```python
from build123d import *

# Parameters (mm, degrees)
SKETCH1_R           = 5
SKETCH1_R_2         = 1.740677898
BOSS_EXTRUDE1_DEPTH = 6
SKETCH2_R           = 1.25
CUT_EXTRUDE1_DEPTH  = 11


with BuildPart() as part:
    # Sketch1 → Boss-Extrude1 (new body)
    with BuildSketch(Plane.XY):
        with Locations((-35.04245283, -0.806603774)):
            Circle(SKETCH1_R)
        with Locations((-35.04245283, -0.806603774)):
            Circle(SKETCH1_R_2, mode=Mode.SUBTRACT)
        with BuildLine():
            Line((-16.04245283, 4.193396226), (-35.04245283, 4.193396226))
            ThreePointArc((-35.04245283, 4.193396226), (-31.506918924, 2.728930132), (-30.04245283, -0.806603774))
            ThreePointArc((-30.04245283, -0.806603774), (-31.506918924, -4.34213768), (-35.04245283, -5.806603774))
            Line((-35.04245283, -5.806603774), (-16.04245283, -5.806603774))
            ThreePointArc((-16.04245283, -5.806603774), (-21.04245283, -0.806603774), (-16.04245283, 4.193396226))
        make_face()
        with Locations((-16.04245283, -0.806603774)):
            Circle(SKETCH1_R)
        with Locations((-16.04245283, -0.806603774)):
            Circle(SKETCH1_R_2, mode=Mode.SUBTRACT)
    extrude(amount=BOSS_EXTRUDE1_DEPTH)

    # Sketch2 → Cut-Extrude1 (cut, through all)
    with BuildSketch(Plane(origin=(0, 4.193396226, 0), x_dir=(1, 0, 0), z_dir=(0, 1, 0))):
        with Locations((-16.04245283, -3)):
            Circle(SKETCH2_R)
    extrude(amount=-CUT_EXTRUDE1_DEPTH, mode=Mode.SUBTRACT)


solid = part.part
```
Can you work these out from the model? Positions are in its coordinate system, mm. Give positions to 0.01 mm unless a question says otherwise; leave off trailing zeros. Order: outer loops, then holes, each group sorted by start corner. A loop starts at its lowest first (then second) coordinate and runs counter-clockwise, first axis right, second up. Notation, with made-up numbers: M -28,31 L 7,31 A20 ccw 7,62 Z; hole C 22,31 d1. An arc over 180 degrees is marked long. Write item = value, one per line. Start each with the question number.
Q1. Suppose I cut it at A-A (z = 3). Write out the boundary of the cut face in (x, y), plus the area to 3 significant figures.
Q2. Suppose I cut it at B-B (x = -15.5). Write out the boundary of the cut face in (y, z), plus the area to 3 significant figures.
Q3. Suppose I cut it at D-D (y = -4.75). Write out the boundary of the cut face in (x, z).
Q4. Suppose I cut it at C-C (z = 1). Write out the boundary of the cut face in (x, y).
Q5. We'd pull the mould along X, two halves only. Please class faces 1 (the cylindrical face through (-11.044, -0.917, 2.958)), 2 (the flat face through (-25, 4.193, 3)), 3 (the cylindrical face through (-17.78, -0.73, 2.96)): pulls with the +X half, pulls with the -X half, needs draft (parallel to the pull), parting line crosses it, or undercut.
Q6. I need wall thicknesses on probe 1 along X at (y, z) = (-0.75, 4.75); probe 2 along X at (y, z) = (0.5, 3.25); probe 3 along Y at (x, z) = (-35, 5). Which ranges of each line are inside material? Lowest first, please. Write a range as [from, to].
Q7. Will these pins go through, and if not, where does the flat tip stop? pin 1 Ø2 at (y, z) = (2.5, 3.5) entering from -X; pin 2 Ø2 at (x, y) = (-35.04, -0.81) entering from -Z.
Check result:
q1.outline = M -35.04,-5.81 L -17.29,-5.81 L -17.29,-2.02 A1.74 cw -17.29,0.4 L -17.29,4.19 L -35.04,4.19 A5 ccw Z; M -14.79,-5.65 A5 ccw -14.79,4.03 L -14.79,0.4 A1.74 cw -14.79,-2.02 Z; hole C -35.04,-0.81 d3.48
q1.area = 233 mm2
q2.outline = M -5.78,0 L -2.46,0 L -2.46,1.87 L -5.78,1.87 Z; M -5.78,4.13 L -2.46,4.13 L -2.46,6 L -5.78,6 Z; M 0.85,0 L 4.16,0 L 4.16,1.87 L 0.85,1.87 Z; M 0.85,4.13 L 4.16,4.13 L 4.16,6 L 0.85,6 Z
q2.area = 24.9 mm2
q3.outline = M -38.12,0 L -12.97,0 L -12.97,6 L -38.12,6 Z; hole C -16.04,3 d2.5
q4.outline = M -35.04,-5.81 L -16.04,-5.81 A5 ccw -16.04,4.19 L -35.04,4.19 A5 ccw Z; hole C -35.04,-0.81 d3.48; hole C -16.04,-0.81 d3.48
q5.face_1 = pulls with the +X half
q5.face_2 = needs draft
q5.face_3 = undercut
q6.probe_1 = [-40.04, -36.78], [-33.3, -17.78], [-14.3, -11.04]
q6.probe_2 = [-39.87, -36.19], [-33.89, -17.27], [-14.82, -11.22]
q6.probe_3 = [-5.81, -2.55], [0.93, 4.19]
q7.pin_1 = -39.48
q7.pin_2 = through
